The listing builds one solid part. Answer for the finished solid, in the listing's coordinates (mm). Face numbers are marked on the shaded views. A direction names the side the tool comes from. Coordinates: 2 decimals unless noted, no trailing zeros. Order: outer loops, then holes, each group sorted by start corner. A loop starts at its lowest first (then second) coordinate and runs counter-clockwise, first axis right, second up. Notation, with made-up numbers: (-5, -30) -> (0, -30) arc R9 cw to (0, -13) -> close; hole circle Ø10 at (34.25, -33). An arc over 180 degrees is marked (long way). One line per question, with ' | ' between items.
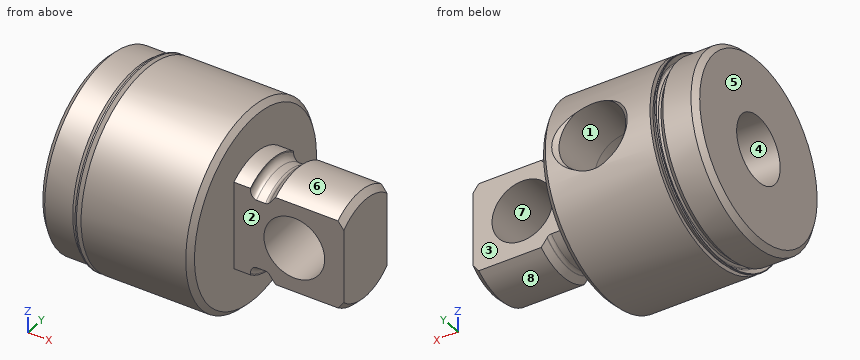
Autodesk Inventor part; units mm, degrees
ref_plane "1_XY" through (24.6126, 0, 0) normal (1, 0, 0) x (0, 0, -1)
ref_plane "1_YZ" through (24.6126, 0, 0) normal (0, 0, -1) x (0, 1, 0)
ref_plane "1_ZX" through (24.6126, 0, 0) normal (0, 1, 0) x (1, 0, 0)
sketch "Sketch_18" plane through (0, 0, 0) normal (0, 0, 1) x (1, 0, 0)
  line L0 (22.225, 0) -> (0, 0)
  line L1 (0, 0) -> (0, 12.846)
  line L2 (0, 12.846) -> (0.762, 13.608)
  line L3 (0.762, 13.608) -> (4.826, 13.608)
  line L4 (4.826, 13.608) -> (5.588, 12.846)
  line L5 (5.588, 12.846) -> (6.35, 12.846)
  line L6 (6.35, 12.846) -> (6.35, 14.1097)
  line L7 (6.35, 14.1097) -> (21.463, 14.1097)
  line L8 (21.463, 14.1097) -> (22.225, 13.3477)
  line L9 (22.225, 13.3477) -> (22.225, 0)
  line L10 (22.225, 0) -> (0, 0)
revolve "Revolution1" add sketch "Sketch_18" angle 360 about axis through (22.225, 0, 0) along (1, 0, 0)
sketch "Sketch_15" plane through (0, 0, 0) normal (0, 0, 1) x (1, 0, 0)
  line L0 (38.1, 0) -> (22.225, 0)
  line L1 (22.225, 0) -> (22.225, 7.9057)
  line L2 (22.225, 7.9057) -> (24.6126, 7.9057)
  line L3 (24.6126, 7.9057) -> (24.6126, 7.7279)
  arc A0 (24.6126, 7.7279) -> (25.5016, 6.839) centre (25.5016, 7.7279) ccw
  line L4 (25.5016, 6.839) -> (26.7843, 6.839)
  arc A1 (26.7843, 6.839) -> (27.383, 7.0708) centre (26.7843, 7.7279) ccw
  line L5 (27.383, 7.0708) -> (27.4129, 7.098)
  line L6 (27.4129, 7.098) -> (28.2524, 7.9375)
  line L7 (28.2524, 7.9375) -> (37.2605, 7.9375)
  line L8 (37.2605, 7.9375) -> (38.1, 7.098)
  line L9 (38.1, 7.098) -> (38.1, 0)
  line L10 (38.1, 0) -> (22.225, 0)
revolve "Revolution2" add sketch "Sketch_15" angle 360 about axis through (38.1, 0, 0) along (1, 0, 0)
thread "Thread1"
sketch "Sketch_70" plane through (38.1, 0, 0) normal (1, 0, 0) x (0, 0, -1)
  line L0 (-56.4388, -28.2194) -> (56.4388, -28.2194)
  line L1 (56.4388, -28.2194) -> (56.4388, 28.2194)
  line L2 (56.4388, 28.2194) -> (-56.4388, 28.2194)
  line L3 (-56.4388, 28.2194) -> (-56.4388, -28.2194)
  line L4 (-28.2194, -4.7308) -> (28.2194, -4.7308)
  line L5 (28.2194, -4.7308) -> (28.2194, 4.7308)
  line L6 (28.2194, 4.7308) -> (-28.2194, 4.7308)
  line L7 (-28.2194, 4.7308) -> (-28.2194, -4.7308)
extrude "Extrusion1" cut sketch "Sketch_70" against normal blind 15.875
sketch "Sketch4" plane through (0, 0, 0) normal (-1, 0, 0) x (0, 0, 1)
  point P0 (0, 0)
hole "Hole1" at (0, 0, 0) direction (1, 0, 0) diameter 9.525 depth 20.955 tip angle 120
sketch "Sketch_47" plane through (0, 0, 0) normal (0, 0, 1) x (1, 0, 0)
  line L0 (15.0876, 0) -> (15.0876, 14.1097)
  line L1 (15.0876, 14.1097) -> (20.5423, 14.1097)
  line L2 (20.5423, 14.1097) -> (19.9073, 13.4747)
  line L3 (19.9073, 13.4747) -> (19.6754, 6.0491)
  line L4 (19.6754, 6.0491) -> (19.6754, 0)
  line L5 (19.6754, 0) -> (15.0876, 0)
  line L6 (15.0876, 0) -> (15.0876, 14.1097)
revolve "Revolution3" cut sketch "Sketch_47" angle 360 about axis through (15.0876, 0, 0) along (0, -1, 0)
thread "Thread2"
sketch "Sketch_24" plane through (0, 0, 0) normal (0, 0, 1) x (1, 0, 0)
  line L0 (6.35, 0) -> (5.588, 0)
  line L1 (5.4861, 14.1097) -> (5.4861, 14.0255)
  line L2 (5.4861, 14.0255) -> (6.2275, 13.2842)
  arc A0 (6.2275, 13.1046) -> (6.2275, 13.2842) centre (6.1377, 13.1944) ccw
  line L3 (6.2275, 13.1046) -> (5.969, 12.846)
  line L4 (5.969, 12.846) -> (5.588, 12.846)
  line L5 (5.588, 12.846) -> (5.588, 12.5921)
  line L6 (5.588, 12.5921) -> (6.35, 12.5921)
  line L7 (6.35, 12.5921) -> (6.35, 13.449)
  line L8 (6.35, 13.449) -> (5.6893, 14.1097)
  line L9 (5.6893, 14.1097) -> (5.4861, 14.1097)
revolve "Revolution4" add sketch "Sketch_24" angle 360 about axis through (6.35, 0, 0) along (1, 0, 0)
sketch "Sketch_43" plane through (0, 0, 0) normal (0, 1, 0) x (-1, 0, 0)
  circle A0 centre (-30.9626, 0) radius 4.3878
extrude "Extrusion2" cut sketch "Sketch_43" along normal mid plane 14.1922
ref_plane "1_XY" through (24.6126, 0, 0) normal (1, 0, 0) x (0, 0, -1)
ref_plane "1_YZ" through (24.6126, 0, 0) normal (0, 0, -1) x (0, 1, 0)
ref_plane "1_ZX" through (24.6126, 0, 0) normal (0, 1, 0) x (1, 0, 0)
ref_plane "c1_XY" through (22.225, 7.9057, 0) normal (0, 0, 1) x (1, 0, 0)
ref_plane "c1_YZ" through (22.225, 7.9057, 0) normal (1, 0, 0) x (0, 1, 0)
ref_plane "c1_ZX" through (22.225, 7.9057, 0) normal (0, 1, 0) x (0, 0, 1)
ref_plane "c2_XY" through (22.225, -7.9057, 0) normal (0, 0, 1) x (1, 0, 0)
ref_plane "c2_YZ" through (22.225, -7.9057, 0) normal (1, 0, 0) x (0, 1, 0)
ref_plane "c2_ZX" through (22.225, -7.9057, 0) normal (0, 1, 0) x (0, 0, 1)
ref_plane "cc1_XY" through (22.225, 0, 0) normal (0, 0, 1) x (1, 0, 0)
ref_plane "cc1_YZ" through (22.225, 0, 0) normal (1, 0, 0) x (0, 1, 0)
ref_plane "cc1_ZX" through (22.225, 0, 0) normal (0, 1, 0) x (0, 0, 1)
ref_plane "cc2_XY" through (24.6126, 0, 0) normal (0, 0, 1) x (1, 0, 0)
ref_plane "cc2_YZ" through (24.6126, 0, 0) normal (1, 0, 0) x (0, 1, 0)
ref_plane "cc2_ZX" through (24.6126, 0, 0) normal (0, 1, 0) x (0, 0, 1)
ref_plane "lovra1_XY" through (33.3248, 0, 0) normal (1, 0, 0) x (0, 0, -1)
ref_plane "lovra1_YZ" through (33.3248, 0, 0) normal (0, 0, -1) x (0, 1, 0)
ref_plane "lovra1_ZX" through (33.3248, 0, 0) normal (0, 1, 0) x (1, 0, 0)
ref_plane "lovra2_XY" through (33.3248, 11.049, 0) normal (1, 0, 0) x (0, 0, -1)
ref_plane "lovra2_YZ" through (33.3248, 11.049, 0) normal (0, 0, -1) x (0, 1, 0)
ref_plane "lovra2_ZX" through (33.3248, 11.049, 0) normal (0, 1, 0) x (1, 0, 0)
ref_plane "lovra21_XY" through (0, 0, 5.2705) normal (1, 0, 0) x (0, 0, -1)
ref_plane "lovra21_YZ" through (0, 0, 5.2705) normal (0, 0, -1) x (0, 1, 0)
ref_plane "lovra21_ZX" through (0, 0, 5.2705) normal (0, 1, 0) x (1, 0, 0)
ref_plane "lovra22_XY" through (0, 0, -5.2705) normal (1, 0, 0) x (0, 0, -1)
ref_plane "lovra22_YZ" through (0, 0, -5.2705) normal (0, 0, -1) x (0, 1, 0)
ref_plane "lovra22_ZX" through (0, 0, -5.2705) normal (0, 1, 0) x (1, 0, 0)
ref_plane "lovra3_XY" through (33.3248, -11.049, 0) normal (1, 0, 0) x (0, 0, -1)
ref_plane "lovra3_YZ" through (33.3248, -11.049, 0) normal (0, 0, -1) x (0, 1, 0)
ref_plane "lovra3_ZX" through (33.3248, -11.049, 0) normal (0, 1, 0) x (1, 0, 0)
ref_plane "olen_XY" through (30.9626, 0, 0) normal (1, 0, 0) x (0, 0, -1)
ref_plane "olen_YZ" through (30.9626, 0, 0) normal (0, 0, -1) x (0, 1, 0)
ref_plane "olen_ZX" through (30.9626, 0, 0) normal (0, 1, 0) x (1, 0, 0)
ref_plane "p1_XY" through (38.1, 0, 4.7308) normal (1, 0, 0) x (0, 0, -1)
ref_plane "p1_YZ" through (38.1, 0, 4.7308) normal (0, 0, -1) x (0, 1, 0)
ref_plane "p1_ZX" through (38.1, 0, 4.7308) normal (0, 1, 0) x (1, 0, 0)
ref_plane "p2_XY" through (38.1, 0, -4.7308) normal (1, 0, 0) x (0, 0, -1)
ref_plane "p2_YZ" through (38.1, 0, -4.7308) normal (0, 0, -1) x (0, 1, 0)
ref_plane "p2_ZX" through (38.1, 0, -4.7308) normal (0, 1, 0) x (1, 0, 0)
ref_plane "port_XY" through (15.0876, 0, 0) normal (0, 0, 1) x (1, 0, 0)
ref_plane "port_YZ" through (15.0876, 0, 0) normal (1, 0, 0) x (0, 1, 0)
ref_plane "port_ZX" through (15.0876, 0, 0) normal (0, 1, 0) x (0, 0, 1)
ref_plane "port2_XY" through (38.1, 0, 0) normal (1, 0, 0) x (0, 0, -1)
ref_plane "port2_YZ" through (38.1, 0, 0) normal (0, 0, -1) x (0, 1, 0)
ref_plane "port2_ZX" through (38.1, 0, 0) normal (0, 1, 0) x (1, 0, 0)
ref_plane "thd1_XY" through (38.1, 0, 7.9375) normal (1, 0, 0) x (0, 0, -1)
ref_plane "thd1_YZ" through (38.1, 0, 7.9375) normal (0, 0, -1) x (0, 1, 0)
ref_plane "thd1_ZX" through (38.1, 0, 7.9375) normal (0, 1, 0) x (1, 0, 0)
ref_plane "thd2_XY" through (38.1, 0, -7.9375) normal (1, 0, 0) x (0, 0, -1)
ref_plane "thd2_YZ" through (38.1, 0, -7.9375) normal (0, 0, -1) x (0, 1, 0)
ref_plane "thd2_ZX" through (38.1, 0, -7.9375) normal (0, 1, 0) x (1, 0, 0)
ref_plane "to_mounting_bracket_XY" through (22.225, 0, 0) normal (1, 0, 0) x (0, 0, -1)
ref_plane "to_mounting_bracket_YZ" through (22.225, 0, 0) normal (0, 0, -1) x (0, 1, 0)
ref_plane "to_mounting_bracket_ZX" through (22.225, 0, 0) normal (0, 1, 0) x (1, 0, 0)
ref_plane "to_nut_XY" through (24.6126, 0, 0) normal (1, 0, 0) x (0, 0, -1)
ref_plane "to_nut_YZ" through (24.6126, 0, 0) normal (0, 0, -1) x (0, 1, 0)
ref_plane "to_nut_ZX" through (24.6126, 0, 0) normal (0, 1, 0) x (1, 0, 0)
ref_plane "to_pin_XY" through (30.9626, 0, 0) normal (0, 1, 0) x (1, 0, 0)
ref_plane "to_pin_YZ" through (30.9626, 0, 0) normal (1, 0, 0) x (0, 0, -1)
ref_plane "to_pin_ZX" through (30.9626, 0, 0) normal (0, 0, -1) x (0, 1, 0)
ref_plane "to_pin_1_XY" through (30.9626, 0, 0) normal (0, 0, 1) x (1, 0, 0)
ref_plane "to_pin_1_YZ" through (30.9626, 0, 0) normal (1, 0, 0) x (0, 1, 0)
ref_plane "to_pin_1_ZX" through (30.9626, 0, 0) normal (0, 1, 0) x (0, 0, 1)
ref_plane "to_pin_r_XY" through (30.9626, 0, 0) normal (0, 0, 1) x (1, 0, 0)
ref_plane "to_pin_r_YZ" through (30.9626, 0, 0) normal (1, 0, 0) x (0, 1, 0)
ref_plane "to_pin_r_ZX" through (30.9626, 0, 0) normal (0, 1, 0) x (0, 0, 1)
ref_plane "to_screw_XY" through (15.0876, 10.2743, -7.0612) normal (0, 1, 0) x (1, 0, 0)
ref_plane "to_screw_YZ" through (15.0876, 10.2743, -7.0612) normal (1, 0, 0) x (0, 0, -1)
ref_plane "to_screw_ZX" through (15.0876, 10.2743, -7.0612) normal (0, 0, -1) x (0, 1, 0)
ref_plane "to_tube_XY" through (5.588, 0, 0) normal (1, 0, 0) x (0, 0, -1)
ref_plane "to_tube_YZ" through (5.588, 0, 0) normal (0, 0, -1) x (0, 1, 0)
ref_plane "to_tube_ZX" through (5.588, 0, 0) normal (0, 1, 0) x (1, 0, 0)
properties part number "09P0Y000_rear_head"
Item 1: Each of these flat-tipped pins is pushed along its axis until it touches: pin 1 Ø1.5 at (x, y) = (9, -10) entering from -Z; pin 2 Ø6 at (x, z) = (21, 2.5) entering from -Y; pin 3 Ø2 at (x, y) = (23.5, -4) entering from -Z; pin 4 Ø3 at (x, y) = (8, -8) entering from +Z. Where does it stop, or does it pass through?
Computed values:
pin 1: stops at z = -10.65 | pin 2: stops at y = -14.11 | pin 3: stops at z = -7.31 | pin 4: stops at z = 12.52
Item 2: For the marked faces 1, 2, 3 and 4, determine the directions among +Z, -Z, +X, -X, +Y, -Y from which every point of the face is accessible in a straight line to the end or side of a thin tool.
Computed values:
face 1: +Y | face 2: +Z, -Z, +X, -Y | face 3: +Z, -Z, +X, +Y | face 4: -X
Item 3: Section B-B, the plane z = 2 is taken. Count the separate pieces of the cut face and the enclosed holes in it, plus the area to 3 significant figures.
Computed values:
separate pieces: 3 | enclosed holes: 0 | area: 417 mm^2
Item 4: Section A-A, the plane x = 2.5 is taken. Give the vertices of the cut face in (y, z) (1 decimal).
Computed values:
outline: circle Ø27.2 at (0, 0); hole circle Ø9.5 at (0, 0)
Item 5: Determine the mould class of the marked faces 5, 6, 7 and 8 for opening direction Z: pulls with the +Z half, pulls with the -Z half, needs draft (parallel to the pull), parting line crosses it, or undercut.
Computed values:
face 5: needs draft | face 6: pulls with the +Z half | face 7: undercut | face 8: pulls with the -Z half
Item 6: Find the intervals of material crossed by L1, parallel to Z at x = 16, y = 0; L2, parallel to Z at x = 6, y = 8; L3, parallel to Y at x = 6, z = -0.25, in increasing order.
Computed values:
L1: z = -14.11 to -4.76, 4.76 to 14.11 | L2: z = -11.24 to -10.89, -10.09 to 10.09, 10.89 to 11.24 | L3: y = -13.8 to -13.51, -12.87 to -4.76, 4.76 to 12.87, 13.51 to 13.8
